```python
from build123d import *

# Parameters (mm, degrees)
SKETCH1_W             = 90
SKETCH1_H             = 55
BOSS_EXTRUDE1_DEPTH   = 5
SKETCH2_W             = 35
SKETCH2_H             = 55
BOSS_EXTRUDE2_DEPTH   = 30
F_1_0MM_DOWEL_HOLE1_D = 14
SKETCH5_W             = 10
SKETCH5_H             = 55
BOSS_EXTRUDE4_DEPTH   = 20
SKETCH8_W             = 20
SKETCH8_H             = 15
BOSS_EXTRUDE5_DEPTH   = 20
CHAMFER1_SIZE2        = 40
CHAMFER1_SIZE         = 19.943264322
SKETCH9_W             = 25
SKETCH9_H             = 55
BOSS_EXTRUDE6_DEPTH   = 7
BOSS_EXTRUDE7_DEPTH   = 55
SKETCH16_W            = 25
SKETCH16_H            = 18
BOSS_EXTRUDE8_DEPTH   = 43
SKETCH17_W            = 25
SKETCH17_H            = 18
CUT_EXTRUDE1_DEPTH    = 43
F_1_0MM_DOWEL_HOLE2_D = 14


with BuildPart() as part:
    # Sketch1 → Boss-Extrude1 (new body)
    with BuildSketch(Plane(origin=(0, 0, 0), x_dir=(1, 0, 0), z_dir=(0, 1, 0))):
        with Locations((45, -27.5)):
            Rectangle(SKETCH1_W, SKETCH1_H)
    extrude(amount=BOSS_EXTRUDE1_DEPTH)

    # Sketch2 → Boss-Extrude2 (add)
    with BuildSketch(Plane(origin=(0, 5, 0), x_dir=(1, 0, 0), z_dir=(0, 1, 0))):
        with Locations((17.5, -27.5)):
            Rectangle(SKETCH2_W, SKETCH2_H)
    extrude(amount=BOSS_EXTRUDE2_DEPTH)

    # Ø1.0mm Dowel Hole1 (through all)
    with Locations(Plane.XY.offset(55)):
        with Locations((20, 20)):
            Hole(F_1_0MM_DOWEL_HOLE1_D / 2)

    # Sketch5 → Boss-Extrude4 (add)
    with BuildSketch(Plane(origin=(0, 5, 0), x_dir=(1, 0, 0), z_dir=(0, 1, 0))):
        with Locations((65, -27.5)):
            Rectangle(SKETCH5_W, SKETCH5_H)
    extrude(amount=BOSS_EXTRUDE4_DEPTH)

    # Sketch8 → Boss-Extrude5 (add)
    with BuildSketch(Plane(origin=(0, 5, 0), x_dir=(1, 0, 0), z_dir=(0, 1, 0))):
        with Locations((80, -7.5)):
            Rectangle(SKETCH8_W, SKETCH8_H)
    extrude(amount=BOSS_EXTRUDE5_DEPTH)

    # Chamfer1
    chamfer1_edges = [part.edges().sort_by_distance(p)[0] for p in [
        (80, 5, 15),
    ]]
    chamfer1_side = [part.faces().sort_by_distance(p)[0] for p in [
        (80, 5.398865286, 15),
    ]]
    chamfer(chamfer1_edges, length=CHAMFER1_SIZE - 0.0001, length2=CHAMFER1_SIZE2 - 0.0001, reference=chamfer1_side[0])  # a hair under: the kernel refuses the full size

    # Sketch9 → Boss-Extrude6 (add)
    with BuildSketch(Plane(origin=(0, 5, 0), x_dir=(1, 0, 0), z_dir=(0, 1, 0))):
        with Locations((47.5, -27.5)):
            Rectangle(SKETCH9_W, SKETCH9_H)
    extrude(amount=BOSS_EXTRUDE6_DEPTH)

    # Sketch12 → Boss-Extrude7 (add)
    with BuildSketch(Plane.XY.offset(55)):
        Polygon((0, 35), (20, 60), (35, 35), (35, 12), (60, 12), (60, 25), (70, 25), (70, 5), (90, 5), (90, 0), (0, 0), align=None)
    extrude(amount=-BOSS_EXTRUDE7_DEPTH)

    # Sketch16 → Boss-Extrude8 (add)
    with BuildSketch(Plane.ZY):
        with Locations((27.5, 51)):
            Rectangle(SKETCH16_W, SKETCH16_H)
    extrude(amount=-BOSS_EXTRUDE8_DEPTH)

    # Sketch17 → Cut-Extrude1 (cut)
    with BuildSketch(Plane.ZY):
        with Locations((27.5, 51)):
            Rectangle(SKETCH17_W, SKETCH17_H)
    extrude(amount=-CUT_EXTRUDE1_DEPTH, mode=Mode.SUBTRACT)

    # Ø1.0mm Dowel Hole2 (through all)
    with Locations(Plane.XY.offset(55)):
        with Locations((20, 20)):
            Hole(F_1_0MM_DOWEL_HOLE2_D / 2)


solid = part.part
```
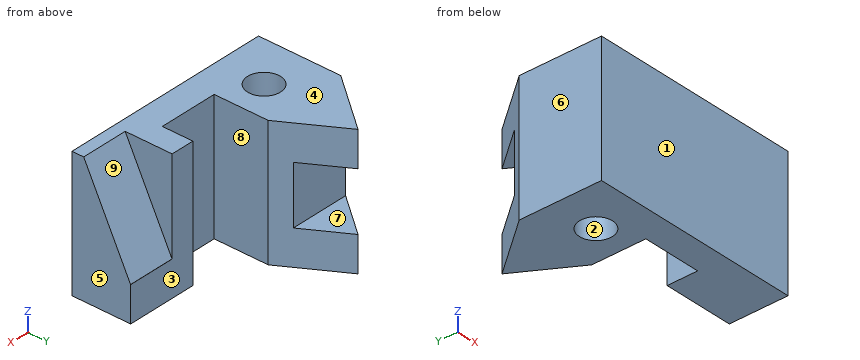
Check sheet for the modelled part. Datum: model origin and axes. Units: mm. Face numbers are marked on the shaded views. A direction names the side the tool comes from. Coordinates: 2 decimals unless noted, no trailing zeros. Write each loop counter-clockwise with the first axis right and the second up, starting at its lowest first coordinate (ties: lowest second). Pieces come first, ordered by that corner, then holes. Notation, with made-up numbers: M 36,75.5 L 57,75.5 A13 ccw 57,100.5 Z; hole C 89.5,-27.75 d2. An arc over 180 degrees is marked long. Write item = value, one per line. Start each with the question number.
1. Mould release check, pull along Y, two halves, no side actions. Record for the marked faces 1, 2, 3 and 4: pulls with the +Y half, pulls with the -Y half, needs draft (parallel to the pull), parting line crosses it, or undercut.
2. Sectioned sample at D-D (z = 22). Record the cut outline in (x, y), then the cut area to 3 significant figures.
3. Tool access check on the marked faces 5, 6, 7, 8 and 9. Record the directions out of +Z, -Z, +X, -X, +Y, -Y that give a thin tool (end or side, any length) a straight path to the whole face; none if there is none.
4. Go/stop test with flat-tipped pins: pin 1 (2 mm diameter, centred on x = 16.5, y = 24.5, fed in from -Z); pin 2 (3 mm diameter, centred on x = 26.5, z = 10.5, fed in from +Y); pin 3 (7.5 mm diameter, centred on x = 43, z = 32.5, fed in from +Y); pin 4 (2 mm diameter, centred on y = 45, z = 12.5, fed in from -X). Record where each tip stops, or that it passes through.
5. Sectioned sample at C-C (x = 22.5). Record the cut outline in (y, z).
6. Thickness scan on probe 1 along X at (y, z) = (20.5, 21); probe 2 along X at (y, z) = (21, 41); probe 3 along Y at (x, z) = (20, 17). Record the ranges inside material, lowest first.
7. Sectioned sample at B-B (y = 23.5). Record the cut outline in (x, z), then the cut area to 3 significant figures.
8. Sectioned sample at A-A (z = 11). Record the cut outline in (x, y).
The answers:
q1.face_1 = pulls with the -Y half
q1.face_2 = undercut
q1.face_3 = pulls with the +Y half
q1.face_4 = needs draft
q2.outline = M 0,0 L 90,0 L 90,21.45 L 70,21.45 L 70,25 L 60,25 L 60,12 L 35,12 L 35,35 L 30.8,42 L 5.6,42 L 0,35 Z; hole C 20,20 d14
q2.area = 2,260 mm²
q3.face_5 = +Z, -Z, +X, +Y, -Y
q3.face_6 = +Z, -Z, -X, +Y, -Y
q3.face_7 = +X, -X, +Y
q3.face_8 = +Z, -Z, +Y
q3.face_9 = +Z, +X, +Y
q4.pin_1 = through
q4.pin_2 = 51.67
q4.pin_3 = 12
q4.pin_4 = 7.2
q5.outline = M 0,0 L 13.46,0 L 13.46,55 L 0,55 Z; M 26.54,0 L 55.83,0 L 55.83,15 L 42,15 L 42,40 L 55.83,40 L 55.83,55 L 26.54,55 Z
q6.probe_1 = 0 to 13.02, 26.98 to 35, 60 to 90
q6.probe_2 = 0 to 13.07, 26.93 to 35, 60 to 70
q6.probe_3 = 0 to 13, 27 to 42
q7.outline = M 0,0 L 13.94,0 L 13.94,55 L 0,55 Z; M 26.06,0 L 35,0 L 35,55 L 26.06,55 Z; M 60,0 L 90,0 L 90,17.89 L 70,17.89 L 70,55 L 60,55 Z
q7.area = 2,170 mm²
q8.outline = M 0,0 L 90,0 L 90,25 L 60,25 L 60,12 L 35,12 L 35,35 L 20,60 L 0,35 Z; hole C 20,20 d14
